```python
from build123d import *

# Parameters (mm, degrees)
SKETCH1_W           = 110
SKETCH1_H           = 40
BOSS_EXTRUDE1_DEPTH = 6.5
SKETCH2_R           = 16.125
CUT_EXTRUDE1_DEPTH  = 5.5
FILLET1_R           = 10
SKETCH3_R           = 2.05
CUT_EXTRUDE2_DEPTH  = 59.781374601
CHAMFER1_SIZE       = 0.5


with BuildPart() as part:
    # Sketch1 → Boss-Extrude1 (new body)
    with BuildSketch(Plane.XY):
        Rectangle(SKETCH1_W, SKETCH1_H)
    extrude(amount=BOSS_EXTRUDE1_DEPTH)

    # Sketch2 → Cut-Extrude1 (cut)
    with BuildSketch(Plane.XY.offset(6.5)):
        Circle(SKETCH2_R)
        with Locations((35, 0)):
            Circle(SKETCH2_R)
        with Locations((-35, 0)):
            Circle(SKETCH2_R)
    extrude(amount=-CUT_EXTRUDE1_DEPTH, mode=Mode.SUBTRACT)

    # Fillet1
    fillet1_edges = [part.edges().sort_by_distance(p)[0] for p in [
        (55, -20, 3.25),
        (-55, -20, 3.25),
        (-55, 20, 3.25),
        (55, 20, 3.25),
    ]]
    fillet(fillet1_edges, radius=FILLET1_R)

    # Sketch3 → Cut-Extrude2 (cut, through all)
    with BuildSketch(Plane.XY.offset(1)):
        Circle(SKETCH3_R)
        with Locations((35, 0)):
            Circle(SKETCH3_R)
        with Locations((-35, 0)):
            Circle(SKETCH3_R)
    extrude(amount=-CUT_EXTRUDE2_DEPTH, mode=Mode.SUBTRACT)

    # Chamfer1
    chamfer1_edges = [part.edges().sort_by_distance(p)[0] for p in [
        (-51.125, 0, 6.5),
        (18.875, 0, 6.5),
        (-16.125, 0, 6.5),
        (55, 0, 0),
        (55, 0, 6.5),
        (0, -20, 0),
        (-55, 0, 0),
        (0, 20, 0),
        (-52.071067812, -17.071067812, 0),
        (-52.071067812, 17.071067812, 0),
        (52.071067812, 17.071067812, 0),
        (52.071067812, -17.071067812, 0),
        (0, -20, 6.5),
        (0, 20, 6.5),
        (-55, 0, 6.5),
        (-52.071067812, -17.071067812, 6.5),
        (-52.071067812, 17.071067812, 6.5),
        (52.071067812, 17.071067812, 6.5),
        (52.071067812, -17.071067812, 6.5),
    ]]
    chamfer(chamfer1_edges, length=CHAMFER1_SIZE)


solid = part.part
```
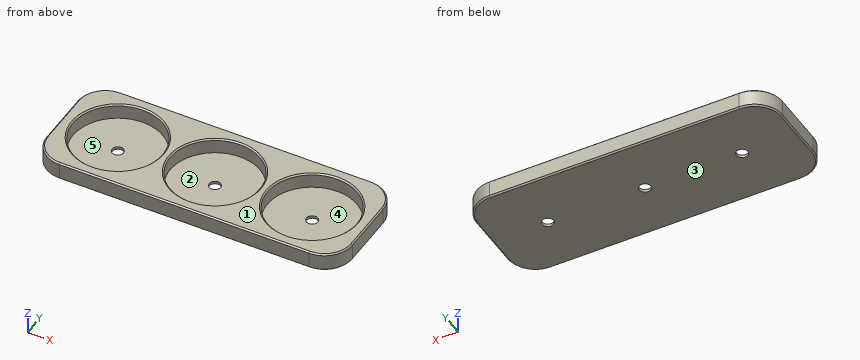
Geometry: final body of the model. Coordinates: model frame, mm. Face numbers are marked on the shaded views. A direction names the side the tool comes from. Round coordinates to 2 decimals unless told otherwise and drop trailing zeros. Order: outer loops, then holes, each group sorted by start corner. A loop starts at its lowest first (then second) coordinate and runs counter-clockwise, first axis right, second up. Notation, with made-up numbers: M 31,17.5 L 71,17.5 A25 cw 71,30.5 Z; hole C -34.75,81.5 d8. An arc over 180 degrees is marked long. One line per item, written item: value.
(1) Pin query (flat end, axial travel): P1, Ø3.5, axis at x = -35, y = 0, coming from the +Z side; P2, Ø19.5, axis at x = 0, y = 0, coming from the -Z side; P3, Ø6, axis at x = -7, y = 7.5, coming from the +Z side. Return the tip coordinate at first contact, or that it passes through.
Result sheet:
P1: through
P2: z = 0
P3: z = 1
(2) Cut plane C-C (y = 0). Give the number of separate pieces and of enclosed holes in the cut face, and give its area (3 significant figures).
Result sheet:
separate pieces: 4
enclosed holes: 0
area: 169 mm2
(3) Cut plane B-B (z = 3.25). Return the cut outline in (x, y) (3 decimals).
Result sheet:
outline: M -55,-10 A10 ccw -45,-20 L 45,-20 A10 ccw 55,-10 L 55,10 A10 ccw 45,20 L -45,20 A10 ccw -55,10 Z; hole C -35,0 d32.25; hole C 0,0 d32.25; hole C 35,0 d32.25
(4) Line query: probe 1 along Y at (x, z) = (-35, 0.5); probe 2 along Y at (x, z) = (0, 3.65) (3 decimals); probe 3 along X at (y, z) = (7, 6.25). Output: solid intervals per line, ascending. Write a range as [from, to].
Result sheet:
probe 1: [-20, -2.05], [2.05, 20]
probe 2: [-20, -16.125], [16.125, 20]
probe 3: [-54.75, -49.8], [-20.2, -14.8], [14.8, 20.2], [49.8, 54.75]
(5) Pull-direction query (Y, two-part tool) for the marked faces 3, 4 and 5; classes: pulls with the +Y half, pulls with the -Y half, needs draft (parallel to the pull), parting line crosses it, or undercut.
Result sheet:
face 3: needs draft
face 4: undercut
face 5: undercut
(6) Cut plane A-A (x = 0). Return the cut outline in (y, z) (3 decimals), and give its area (3 significant figures).
Result sheet:
outline: M -20,0.5 L -19.5,0 L -2.05,0 L -2.05,1 L -16.125,1 L -16.125,6 L -16.625,6.5 L -19.5,6.5 L -20,6 Z; M 2.05,0 L 19.5,0 L 20,0.5 L 20,6 L 19.5,6.5 L 16.625,6.5 L 16.125,6 L 16.125,1 L 2.05,1 Z
area: 77.8 mm2
(7) Reachability of the marked faces 1 and 2 from +Z, -Z, +X, -X, +Y, -Y: full face, straight path, thin tool, end or side. Return the list, or none.
Result sheet:
face 1: +Z, +X, -X, +Y, -Y
face 2: +Z
